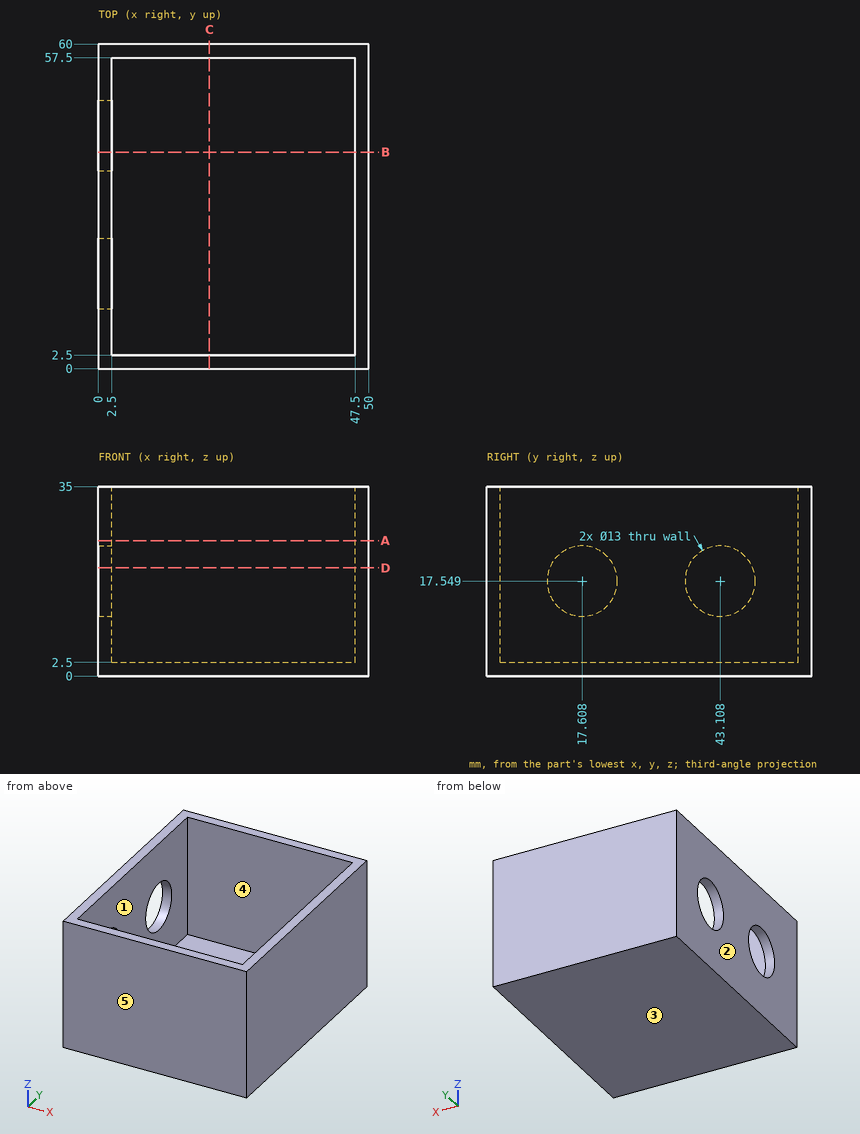
The figure shows three views and two pictorial views of one solid part (mm, origin at its lowest corner). Answer the questions. A direction names the side the tool comes from. Coordinates: 2 decimals unless noted, no trailing zeros. Write each loop counter-clockwise with the first axis right and the second up, starting at its lowest first coordinate (ties: lowest second). Pieces come first, ordered by that corner, then holes. Notation, with made-up numbers: (72.5, 62) -> (106.5, 62) arc R19 cw to (106.5, 71) -> close; hole circle Ø5 at (23.5, 16.25). An arc over 180 degrees is marked (long way). Return JSON: item names as keys, results as strings.
1. A cutting plane is placed at B-B (y = 40). Determine the outline of the cut face in (x, z), and give its area (3 significant figures).
Found:
{"outline": "(0, 0) -> (50, 0) -> (50, 35) -> (47.5, 35) -> (47.5, 2.5) -> (2.5, 2.5) -> (2.5, 11.84) -> (0, 11.84) -> close; (0, 23.26) -> (2.5, 23.26) -> (2.5, 35) -> (0, 35) -> close", "area": "259 mm2"}
2. Determine the mould class of the marked faces 1, 2 and 3 for opening direction X: pulls with the +X half, pulls with the -X half, needs draft (parallel to the pull), parting line crosses it, or undercut.
Found:
{"face 1": "undercut", "face 2": "pulls with the -X half", "face 3": "needs draft"}
3. A cutting plane is placed at D-D (z = 20). Determine the outline of the cut face in (x, y), and give its area (3 significant figures).
Found:
{"outline": "(0, 0) -> (50, 0) -> (50, 60) -> (0, 60) -> (0, 49.13) -> (2.5, 49.13) -> (2.5, 57.5) -> (47.5, 57.5) -> (47.5, 2.5) -> (2.5, 2.5) -> (2.5, 11.59) -> (0, 11.59) -> close; (0, 23.63) -> (2.5, 23.63) -> (2.5, 37.09) -> (0, 37.09) -> close", "area": "465 mm2"}
4. Each of these flat-tipped pins is pushed along its axis until it touches: P1, Ø13.5, axis at x = 36, y = 22.5, coming from the +Z side; P2, Ø2, axis at x = 10.5, y = 27.5, coming from the -Z side. Where does it stop, or does it pass through?
Found:
{"P1": "z = 2.5", "P2": "z = 0"}
5. Find the intervals of material crossed by line 1 along X through (y, z) = (39, 32); line 2 along Y through (x, z) = (3.5, 9.5); line 3 along Z through (x, y) = (11.5, 50), in increasing order. Write a range as from..to.
Found:
{"line 1": "0..2.5, 47.5..50", "line 2": "0..2.5, 57.5..60", "line 3": "0..2.5"}
6. A cutting plane is placed at C-C (x = 20.5). Determine the outline of the cut face in (y, z).
Found:
{"outline": "(0, 0) -> (60, 0) -> (60, 35) -> (57.5, 35) -> (57.5, 2.5) -> (2.5, 2.5) -> (2.5, 35) -> (0, 35) -> close"}
7. A cutting plane is placed at A-A (z = 25). Determine the outline of the cut face in (x, y).
Found:
{"outline": "(0, 0) -> (50, 0) -> (50, 60) -> (0, 60) -> close; hole (2.5, 2.5) -> (47.5, 2.5) -> (47.5, 57.5) -> (2.5, 57.5) -> close"}
8. A tool of negligible diameter and unlimited length cuts with its end or side. For the marked faces 4 and 5, from which of +Z, -Z, +X, -X, +Y, -Y can it reach the whole face along a straight path? Write none if from no direction.
Found:
{"face 4": "+Z", "face 5": "+Z, -Z, +X, -X, -Y"}
